Geometry: see drawing. Coordinates: mm, zero at the bounding-box minimum. A direction names the side the tool comes from. Give positions to 0.01 mm unless a question says otherwise; leave off trailing zeros. Order: outer loops, then holes, each group sorted by start corner. A loop starts at its lowest first (then second) coordinate and runs counter-clockwise, first axis right, second up. Notation, with made-up numbers: M 61.5,-27 L 111.5,-27 A22 cw 111.5,-5 Z; hole C 40.5,-38 d7. An arc over 180 degrees is marked long. Answer as a JSON object with one key per item and string values. Group by question number.
1. Section query D-D (x = 15.5). Output: boundary loops of the cut face in (y, z), plus the area to 3 significant figures.
2. Material intervals for L1, parallel to X at y = 3.55, z = 12.5; L2, parallel to Z at x = 12.51, y = 2.45 (3 decimals); L3, parallel to Z at x = 12.51, y = 0.5, sorted ascending. Write a range as [from, to].
3. Pull-direction query (X, two-part tool) for the marked faces 3, 4 and 5; classes: +X half, -X half, draft (parallel to the pull), parting line (faces both ways), or undercut.
4. Section query A-A (z = 13). Output: boundary loops of the cut face in (x, y).
5. Pin query (flat end, axial travel): P1, Ø1.5, axis at x = 9, z = 6.5, coming from the +Y side; P2, Ø5, axis at x = 13.5, z = 9, coming from the -Y side. Return the tip coordinate at first contact, or that it passes through.
6. Section query C-C (y = 2.45). Output: boundary loops of the cut face in (x, z) (3 decimals).
7. Section query B-B (x = 12.51). Output: boundary loops of the cut face in (y, z) (3 decimals), plus the area to 3 significant figures.
8. Set-up query: the marked faces 1 and 2. Return all of +Z, -Z, +X, -X, +Y, -Y with unobstructed straight access to the full face (end or side cutting, diameter ignored); none if empty.
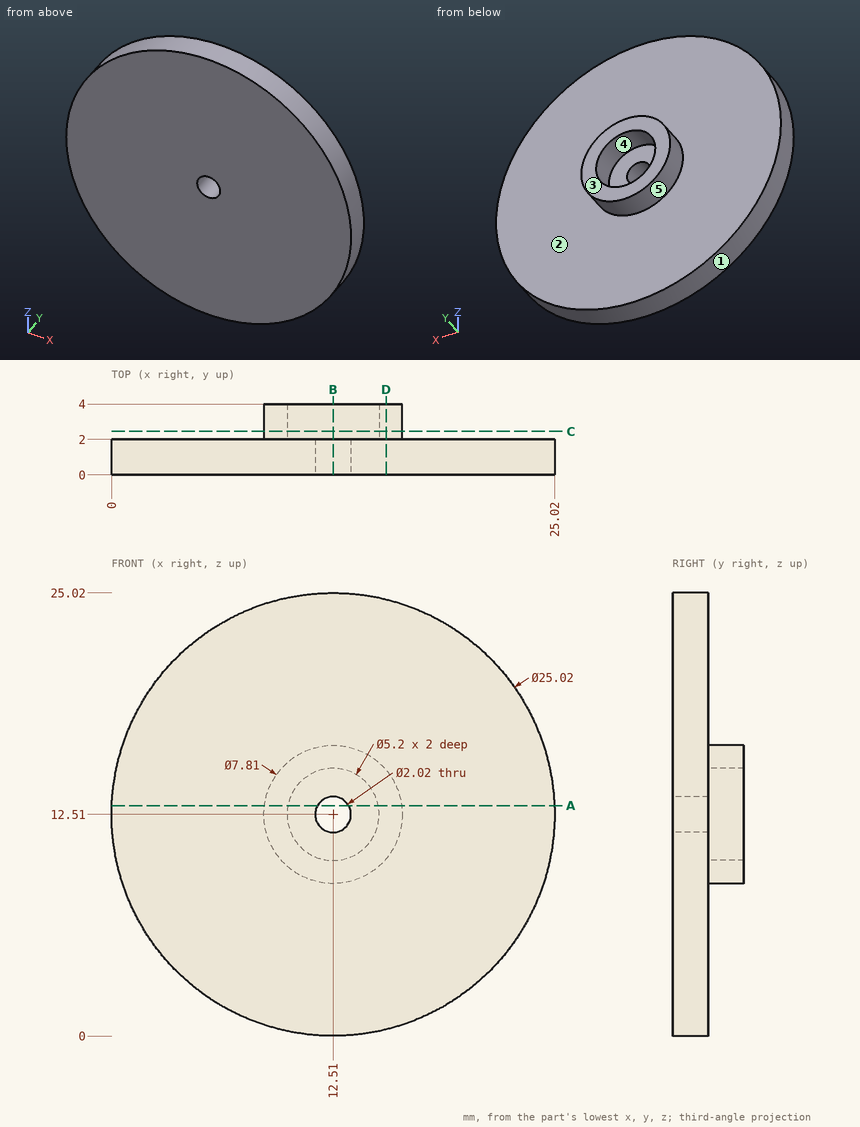
Answer sheet:
{
 "1": {"outline": "M 0,0.36 L 2,0.36 L 2,10 L 4,10 L 4,15.02 L 2,15.02 L 2,24.66 L 0,24.66 Z", "area": "58.6 mm^2"},
 "2": {"L1": "[8.61, 9.91], [15.11, 16.41]", "L2": "[8.605, 9.91], [15.11, 16.415]", "L3": "[0, 11.5], [13.52, 25.02]"},
 "3": {"face 3": "draft", "face 4": "undercut", "face 5": "parting line"},
 "4": {"outline": "M 0.01,0 L 11.63,0 L 11.63,2 L 9.96,2 L 9.96,4 L 8.64,4 L 8.64,2 L 0.01,2 Z; M 13.39,0 L 25.01,0 L 25.01,2 L 16.38,2 L 16.38,4 L 15.06,4 L 15.06,2 L 13.39,2 Z"},
 "5": {"P1": "y = 2", "P2": "y = 0"},
 "6": {"outline": "C 12.51,12.51 d7.81; hole C 12.51,12.51 d5.2"},
 "7": {"outline": "M 0,0 L 2,0 L 2,8.605 L 4,8.605 L 4,9.91 L 2,9.91 L 2,11.5 L 0,11.5 Z; M 0,13.52 L 2,13.52 L 2,15.11 L 4,15.11 L 4,16.415 L 2,16.415 L 2,25.02 L 0,25.02 Z", "area": "51.2 mm^2"},
 "8": {"face 1": "+Y, -Y", "face 2": "+Y"}
}
